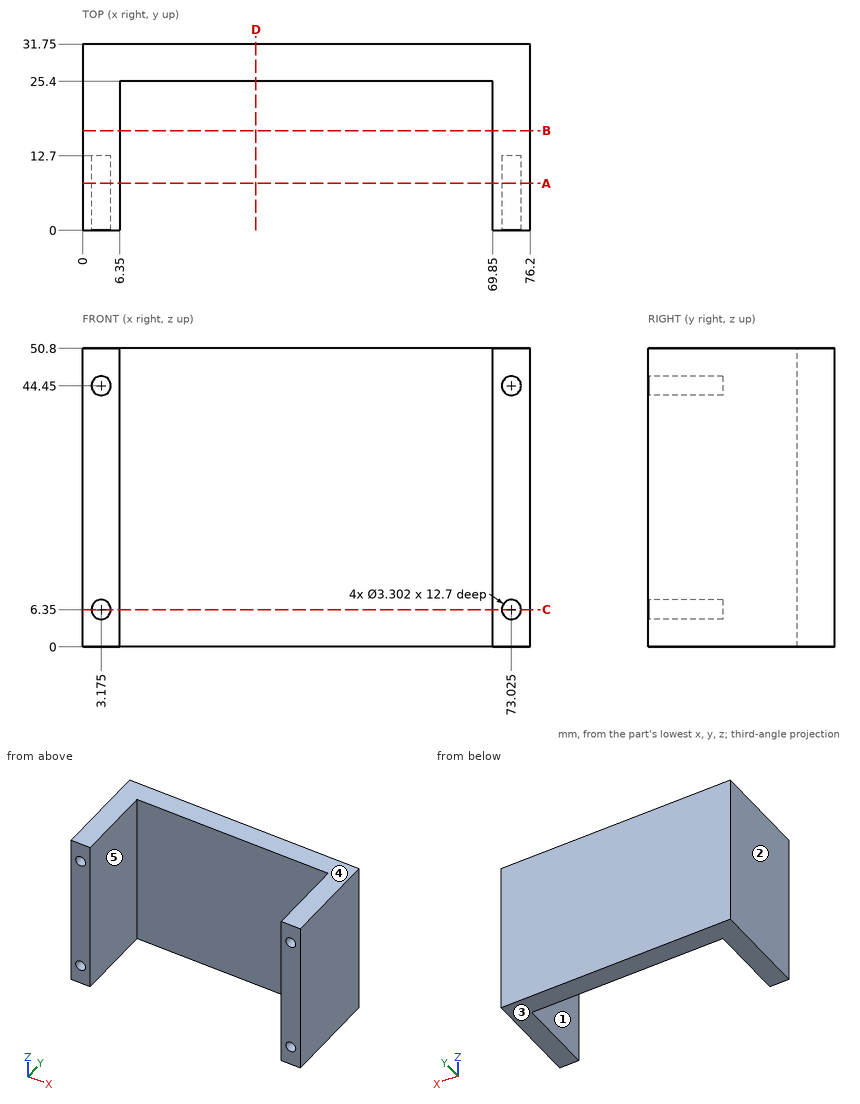
Study the drawing (mm; zero at the part's minimum x, y, z) and answer. A direction names the side the tool comes from. Round coordinates to 2 decimals unless told otherwise and drop trailing zeros. Order: outer loops, then holes, each group sorted by start corner. A loop starts at its lowest first (then second) coordinate and runs counter-clockwise, first axis right, second up. Notation, with made-up numbers: (37, 9) -> (82, 9) arc R10 ccw to (82, 26) -> close; hole circle Ø7 at (43.5, 6.5). An arc over 180 degrees is marked (long way). Answer as CSV lines item,"result". Start each with the question number.
(1) The part is cut by section B-B (y = 17). Determine the outline of the cut face in (x, z).
(2) For a pull along X with two mould halves and no side action, classify the marked faces 1, 2 and 3 as +X half, -X half, draft (parallel to the pull), parting line (faces both ways), or undercut.
(3) The part is cut by section A-A (y = 8). Determine the outline of the cut face in (x, z) (3 decimals), then the cut area to 3 significant figures.
(4) Flat-ended cylindrical pins translate along their axes: pin 1 Ø10 at (x, y) = (55, 21.5) entering from +Z; pin 2 Ø2.5 at (x, z) = (73, 6.5) entering from -Y. Find the tip coordinate at first contact, or state that the pin passes through.
(5) The part is cut by section C-C (z = 6.35). Determine the outline of the cut face in (x, y).
(6) A tool of negligible diameter and unlimited length cuts with its end or side. For the marked faces 4 and 5, from which of +Z, -Z, +X, -X, +Y, -Y can it reach the whole face along a straight path? Write none if from no direction.
(7) Find the intervals of material crossed by probe 1 along X at (y, z) = (6, 34); probe 2 along X at (y, z) = (5, 44); probe 3 along Z at (x, y) = (4, 4), in increasing order. Write a range as from..to.
(8) The part is cut by section D-D (x = 29.5). Determine the outline of the cut face in (y, z).
Evaluation:
1,outline,"(0, 0) -> (6.35, 0) -> (6.35, 50.8) -> (0, 50.8) -> close; (69.85, 0) -> (76.2, 0) -> (76.2, 50.8) -> (69.85, 50.8) -> close"
2,face 1,"undercut"
2,face 2,"-X half"
2,face 3,"draft"
3,outline,"(0, 0) -> (6.35, 0) -> (6.35, 50.8) -> (0, 50.8) -> close; (69.85, 0) -> (76.2, 0) -> (76.2, 50.8) -> (69.85, 50.8) -> close; hole circle Ø3.302 at (3.175, 6.35); hole circle Ø3.302 at (3.175, 44.45); hole circle Ø3.302 at (73.025, 6.35); hole circle Ø3.302 at (73.025, 44.45)"
3,area,"611 mm²"
4,pin 1,"z = 50.8"
4,pin 2,"y = 12.7"
5,outline,"(0, 0) -> (1.52, 0) -> (1.52, 12.7) -> (4.83, 12.7) -> (4.83, 0) -> (6.35, 0) -> (6.35, 25.4) -> (69.85, 25.4) -> (69.85, 0) -> (71.37, 0) -> (71.37, 12.7) -> (74.68, 12.7) -> (74.68, 0) -> (76.2, 0) -> (76.2, 31.75) -> (0, 31.75) -> close"
6,face 4,"+Z, +X, -X, +Y, -Y"
6,face 5,"+Z, -Z, -Y"
7,probe 1,"0..6.35, 69.85..76.2"
7,probe 2,"0..1.59, 4.76..6.35, 69.85..71.44, 74.61..76.2"
7,probe 3,"0..4.92, 7.78..43.02, 45.88..50.8"
8,outline,"(25.4, 0) -> (31.75, 0) -> (31.75, 50.8) -> (25.4, 50.8) -> close"
